Can you work these out from the model? Positions are in its coordinate system, mm. A direction names the side the tool comes from. Coordinates: 2 decimals unless noted, no trailing zeros. Loops run counter-clockwise (first coordinate to the right, second up) from the corner with the lowest first, then second, coordinate; pieces in that order, holes last. Notation, with made-up numbers: (41.5, -32) -> (82.5, -32) arc R10 cw to (82.5, -18) -> close; hole circle Ø5 at (29, -32.75). An arc over 180 degrees is marked (long way). Put each result on its own line as item: value. Start each with the question number.
Item 1: If we section it at A-A on x = 3: Please give me the cut outline in (y, z).
Item 2: If we section it at D-D on y = -0.5: Please give me the cut outline in (x, z), plus the area to 3 significant figures.
Item 3: If we section it at C-C on z = 2.1: Please give me the cut outline in (x, y), plus the area to 3 significant figures.
Item 4: Will these pins go through, and if not, where does the flat tip stop? P1, Ø8, axis at x = 22.45, y = -14.7, coming from the -Z side; P2, Ø6, axis at x = -9, y = -24.5, coming from the -Z side; P3, Ø0.8, axis at y = 21, z = 1.5, coming from the -X side; P4, Ø1, axis at x = -22.5, z = 2, coming from the +Y side.
Item 5: Please list where these lines run through material, in increasing order: L1, parallel to X at y = -2, z = 0.8; L2, parallel to Y at x = -12.5, z = 1.45; L3, parallel to Y at x = -11, z = 1. Write a range as from..to.
Item 6: If we section it at B-B on y = -16: Please give me the cut outline in (x, z), plus the area to 3 significant figures.
Item 7: For faces 1 (the cylindrical face through (-27.35, -3.14, 0.25)), 2 (the flat face through (11.1, 26.1, 1.2)), 3 (the cylindrical face through (2.761, 20.073, 1.232)), 4 (the flat face through (-23, 16.353, 1)), 5 (the cylindrical face through (-5.8, 23.43, 0.49)), which set-ups out of +Z, -Z, +X, -X, +Y, -Y let a thin tool reach every point of the face, with its end or its side?
Item 8: We'd pull the mould along Y, two halves only. Please class faces 6 (the flat face through (22, -28.197, 1)), 7 (the flat face through (4, 28.403, 1)), 8 (the cylindrical face through (20.608, -13.007, 1.486)): pulls with the +Y half, pulls with the -Y half, needs draft (parallel to the pull), parting line crosses it, or undercut.
```python
from build123d import *

# Parameters (mm, degrees)
SKETCH_1_R          = 3
SKETCH_1_R_2        = 2.5
EXTRUDE_1_DEPTH     = 2.5
EXTRUDE_START       = -2
SKETCH_3_R          = 2.5
EXTRUDE_3_DEPTH     = 2
SKETCH_7_R          = 2.65
CUT_EXTRUDE_1_DEPTH = 1
CHAMFER_1_SIZE      = 1
CUT_EXTRUDE_3_REACH = 53.597
SKETCH_10_R         = 2.5
CUT_EXTRUDE_4_REACH = 53.635
CHAMFER_2_SIZE      = 1.5
CUT_EXTRUDE_5_REACH = 53.635
CHAMFER_3_SIZE      = 2
CUT_EXTRUDE_6_REACH = 49.547
SKETCH_15_W         = 9
SKETCH_15_H         = 44.55
SKETCH_15_H_2       = 52
CUT_EXTRUDE_7_REACH = 42.704
SKETCH_16_R         = 2.5
CHAMFER_4_SIZE      = 1.5
SKETCH_17_R         = 2
CUT_EXTRUDE_8_DEPTH = 10


with BuildPart() as part:
    # 스케치1 → 보스-돌출1 (new body)
    with BuildSketch(Plane.XY):
        with BuildLine():
            Line((-27.349187557, -28.196867314), (-7.694270353, -28.196867314))
            Line((-7.694270353, -28.196867314), (-3.192250131, -23.196867314))
            Line((-3.192250131, -23.196867314), (12.267749869, -23.196867314))
            Line((12.267749869, -23.196867314), (17.250812443, -27.683637009))
            Line((17.250812443, -27.683637009), (17.250812443, -14.696867314))
            ThreePointArc((17.250812443, -14.696867314), (22.450812443, -9.496867314), (27.650812443, -14.696867314))
            Line((27.650812443, -14.696867314), (27.650812443, -28.196867314))
            Line((27.650812443, -28.196867314), (40.650812443, -28.196867314))
            Line((40.650812443, -28.196867314), (40.650812443, 12.183132686))
            Line((40.650812443, 12.183132686), (28.992507116, 23.803132686))
            Line((28.992507116, 23.803132686), (13.742507116, 23.803132686))
            Line((13.742507116, 23.803132686), (8.450812443, 28.403132686))
            Line((8.450812443, 28.403132686), (-0.749187557, 28.403132686))
            Line((-0.749187557, 28.403132686), (-5.349187557, 23.803132686))
            Line((-5.349187557, 23.803132686), (-28.149187557, 23.803132686))
            Line((-28.149187557, 23.803132686), (-43.049187557, 8.903132686))
            Line((-43.049187557, 8.903132686), (-43.049187557, -28.196867314))
            Line((-43.049187557, -28.196867314), (-37.749187557, -28.196867314))
            Line((-37.749187557, -28.196867314), (-37.749187557, -3.196867314))
            ThreePointArc((-37.749187557, -3.196867314), (-29.949187557, 1.306464785), (-29.949187557, -7.700199414))
            Line((-29.949187557, -7.700199414), (-29.949187557, -28.196867314))
            Line((-29.949187557, -28.196867314), (-27.349187557, -28.196867314))
        make_face()
        with Locations((8.802507116, -1.986867314)):
            Circle(SKETCH_1_R, mode=Mode.SUBTRACT)
        with Locations((-21.197492884, 7.013132686)):
            Circle(SKETCH_1_R_2, mode=Mode.SUBTRACT)
        with Locations((3.302507116, 22.513132686)):
            Circle(SKETCH_1_R_2, mode=Mode.SUBTRACT)
    extrude(amount=EXTRUDE_1_DEPTH)

    # 스케치3 → 보스-돌출3 (add)
    # profile 1 of 2: a face of its own
    with BuildSketch(Plane.XY.offset(2.5).offset(EXTRUDE_START)):
        with BuildLine():
            Line((27.650812443, -14.696867314), (27.650812443, -28.196867314))
            Line((27.650812443, -28.196867314), (17.764042748, -28.196867314))
            Line((17.764042748, -28.196867314), (17.250812443, -27.683637009))
            Line((17.250812443, -27.683637009), (17.250812443, -14.696867314))
            ThreePointArc((17.250812443, -14.696867314), (22.450812443, -9.496867314), (27.650812443, -14.696867314))
        make_face()
        with Locations((22.450812443, -14.696867314)):
            Circle(SKETCH_3_R, mode=Mode.SUBTRACT)
    # profile 2 of 2: a face of its own
    with BuildSketch(Plane.XY.offset(2.5).offset(EXTRUDE_START)):
        with BuildLine():
            Line((-29.949187557, -7.700199414), (-29.949187557, -28.196867314))
            Line((-29.949187557, -28.196867314), (-30.049187557, -28.196867314))
            Line((-30.049187557, -28.196867314), (-37.749187557, -28.196867314))
            Line((-37.749187557, -28.196867314), (-37.749187557, -3.196867314))
            ThreePointArc((-37.749187557, -3.196867314), (-29.949187557, 1.306464785), (-29.949187557, -7.700199414))
        make_face()
        with Locations((-32.549187557, -3.196867314)):
            Circle(SKETCH_3_R, mode=Mode.SUBTRACT)
    extrude(amount=EXTRUDE_3_DEPTH)

    # 스케치7 → 컷-돌출1 (cut)
    with BuildSketch(Plane(origin=(0, 0, 0), x_dir=(-1, 0, 0), z_dir=(0, 0, -1))):
        with Locations((6.149187557, 20.803132686)):
            Circle(SKETCH_7_R)
        with Locations((8.049187557, -24.196867314)):
            Circle(SKETCH_7_R)
        with BuildLine():
            Line((-26.406412787, 7.908733029), (-32.895212099, 7.908733029))
            ThreePointArc((-32.895212099, 7.908733029), (-33.708384897, 8.245560231), (-34.045212099, 9.058733029))
            Line((-34.045212099, 9.058733029), (-34.045212099, 15.547532342))
            ThreePointArc((-34.045212099, 15.547532342), (-33.708384897, 16.36070514), (-32.895212099, 16.697532342))
            Line((-32.895212099, 16.697532342), (-29.650812443, 16.697532342))
            ThreePointArc((-29.650812443, 16.697532342), (-26.543502647, 15.410442482), (-25.256412787, 12.303132686))
            Line((-25.256412787, 12.303132686), (-25.256412787, 9.058733029))
            ThreePointArc((-25.256412787, 9.058733029), (-25.593239988, 8.245560231), (-26.406412787, 7.908733029))
        make_face()
    extrude(amount=-CUT_EXTRUDE_1_DEPTH, mode=Mode.SUBTRACT)

    # 모따기1
    chamfer_1_edges = [part.edges().sort_by_distance(p)[0] for p in [
        (-43.049187557, -28.196867314, 1.25),
        (40.650812443, -28.196867314, 1.25),
    ]]
    chamfer(chamfer_1_edges, length=CHAMFER_1_SIZE)

    # 스케치10 → 컷-돌출3 (cut, up to next)
    with BuildSketch(Plane(origin=(0, 0, 1), x_dir=(-1, 0, 0), z_dir=(0, 0, -1)), mode=Mode.PRIVATE) as cut_extrude_3_sk1:
        with Locations((-29.650812443, 12.303132686)):
            Circle(SKETCH_10_R)
    cut_extrude_3_tool1 = extrude(cut_extrude_3_sk1.sketch, amount=-CUT_EXTRUDE_3_REACH, mode=Mode.PRIVATE) & part.part
    add(cut_extrude_3_tool1.solids().sort_by_distance((29.650812, 12.303133, 1))[0], mode=Mode.SUBTRACT)

    # 스케치12 → 컷-돌출4 (cut, up to next)
    with BuildSketch(Plane(origin=(0, 0, 0), x_dir=(-1, 0, 0), z_dir=(0, 0, -1)), mode=Mode.PRIVATE) as cut_extrude_4_sk1:
        Polygon((16.749187557, 23.803132686), (16.749187557, 16.353132686), (35.599187557, 16.353132686), (28.149187557, 23.803132686), align=None)
    cut_extrude_4_tool1 = extrude(cut_extrude_4_sk1.sketch, amount=-CUT_EXTRUDE_4_REACH, mode=Mode.PRIVATE) & part.part
    add(cut_extrude_4_tool1.solids().sort_by_distance((-24.464587, 19.772334, 0))[0], mode=Mode.SUBTRACT)

    # 모따기2
    chamfer_2_edges = [part.edges().sort_by_distance(p)[0] for p in [
        (-16.749187557, 23.803132686, 1.25),
        (-16.749187557, 16.353132686, 1.25),
    ]]
    chamfer(chamfer_2_edges, length=CHAMFER_2_SIZE)

    # 스케치13 → 컷-돌출5 (cut, up to next)
    with BuildSketch(Plane(origin=(0, 0, 0), x_dir=(-1, 0, 0), z_dir=(0, 0, -1)), mode=Mode.PRIVATE) as cut_extrude_5_sk1:
        Polygon((-34.689283113, 18.125074406), (-34.689283113, -28.196867314), (-39.650812443, -28.196867314), (-40.650812443, -27.196867314), (-40.650812443, 12.183132686), align=None)
    cut_extrude_5_tool1 = extrude(cut_extrude_5_sk1.sketch, amount=-CUT_EXTRUDE_5_REACH, mode=Mode.PRIVATE) & part.part
    # 스케치13 → 컷-돌출5 (cut, up to next)
    with BuildSketch(Plane(origin=(0, 0, 0), x_dir=(-1, 0, 0), z_dir=(0, 0, -1)), mode=Mode.PRIVATE) as cut_extrude_5_sk2:
        Polygon((38.049187557, 13.903132686), (43.049187557, 8.903132686), (43.049187557, -27.196867314), (42.049187557, -28.196867314), (38.049187557, -28.196867314), align=None)
    cut_extrude_5_tool2 = extrude(cut_extrude_5_sk2.sketch, amount=-CUT_EXTRUDE_5_REACH, mode=Mode.PRIVATE) & part.part
    add(cut_extrude_5_tool1.solids().sort_by_distance((37.59669, -6.446011, 0))[0], mode=Mode.SUBTRACT)
    add(cut_extrude_5_tool2.solids().sort_by_distance((-40.49096, -8.321213, 0))[0], mode=Mode.SUBTRACT)

    # 모따기3
    chamfer_3_edges = [part.edges().sort_by_distance(p)[0] for p in [
        (-38.049187557, -28.196867314, 1.25),
        (34.689283113, -28.196867314, 1.25),
    ]]
    chamfer(chamfer_3_edges, length=CHAMFER_3_SIZE)

    # 스케치15 → 컷-돌출6 (cut, up to next)
    with BuildSketch(Plane.XY.offset(2.5), mode=Mode.PRIVATE) as cut_extrude_6_sk1:
        with Locations((-33.549187557, -5.921867314)):
            Rectangle(SKETCH_15_W, SKETCH_15_H)
    cut_extrude_6_tool1 = extrude(cut_extrude_6_sk1.sketch, amount=-CUT_EXTRUDE_6_REACH, mode=Mode.PRIVATE) & part.part
    # 스케치15 → 컷-돌출6 (cut, up to next)
    with BuildSketch(Plane.XY.offset(2.5), mode=Mode.PRIVATE) as cut_extrude_6_sk2:
        with Locations((30.189283113, -2.196867314)):
            Rectangle(SKETCH_15_W, SKETCH_15_H_2)
    cut_extrude_6_tool2 = extrude(cut_extrude_6_sk2.sketch, amount=-CUT_EXTRUDE_6_REACH, mode=Mode.PRIVATE) & part.part
    add(cut_extrude_6_tool1.solids().sort_by_distance((-33.549188, -5.921867, 2.5))[0], mode=Mode.SUBTRACT)
    add(cut_extrude_6_tool2.solids().sort_by_distance((30.189283, -2.196867, 2.5))[0], mode=Mode.SUBTRACT)

    # 스케치16 → 컷-돌출7 (cut, up to next)
    with BuildSketch(Plane(origin=(0, 0, 0), x_dir=(-1, 0, 0), z_dir=(0, 0, -1)), mode=Mode.PRIVATE) as cut_extrude_7_sk1:
        with Locations((11.549187557, -2.196867314)):
            Circle(SKETCH_16_R)
    cut_extrude_7_tool1 = extrude(cut_extrude_7_sk1.sketch, amount=-CUT_EXTRUDE_7_REACH, mode=Mode.PRIVATE) & part.part
    add(cut_extrude_7_tool1.solids().sort_by_distance((-11.549188, -2.196867, 0))[0], mode=Mode.SUBTRACT)

    # 모따기4
    chamfer_4_edges = [part.edges().sort_by_distance(p)[0] for p in [
        (-29.049187557, 16.353132686, 1.25),
        (-29.049187557, -28.196867314, 1.25),
    ]]
    chamfer(chamfer_4_edges, length=CHAMFER_4_SIZE)

    # 스케치17 → 컷-돌출8 (cut)
    with BuildSketch(Plane(origin=(0, 0, 0), x_dir=(-1, 0, 0), z_dir=(0, 0, -1))):
        with Locations((11.219187557, 20.503132686)):
            Circle(SKETCH_17_R)
    extrude(amount=-CUT_EXTRUDE_8_DEPTH, mode=Mode.SUBTRACT)


solid = part.part
```
Solutions:
1. outline: (-23.2, 0) -> (20.03, 0) -> (20.03, 2.5) -> (-23.2, 2.5) -> close; (24.99, 0) -> (28.4, 0) -> (28.4, 2.5) -> (24.99, 2.5) -> close
2. outline: (-29.05, 0.5) -> (-28.1, 0.5) -> (-28.1, 0) -> (-13.39, 0) -> (-13.39, 2.5) -> (-29.05, 2.5) -> close; (-9.71, 0) -> (6.2, 0) -> (6.2, 2.5) -> (-9.71, 2.5) -> close; (11.41, 0) -> (25.69, 0) -> (25.69, 2.5) -> (11.41, 2.5) -> close
2. area: 114 mm^2
3. outline: (-29.05, -26.7) -> (-27.55, -28.2) -> (-7.69, -28.2) -> (-3.19, -23.2) -> (12.27, -23.2) -> (17.25, -27.68) -> (17.76, -28.2) -> (25.69, -28.2) -> (25.69, 23.8) -> (13.74, 23.8) -> (8.45, 28.4) -> (-0.75, 28.4) -> (-5.35, 23.8) -> (-15.25, 23.8) -> (-16.75, 22.3) -> (-16.75, 17.85) -> (-18.25, 16.35) -> (-27.55, 16.35) -> (-29.05, 14.85) -> close; hole circle Ø5 at (-21.2, 7.01); hole circle Ø5 at (-11.55, -2.2); hole circle Ø4 at (-11.22, 20.5); hole circle Ø5 at (3.3, 22.51); hole circle Ø6 at (8.8, -1.99); hole circle Ø5 at (22.45, -14.7)
3. area: 2,600 mm^2
4. P1: z = 0.5
4. P2: z = 0
4. P3: x = -16.75
4. P4: y = 16.35
5. L1: -29.05..-14.04, -9.06..5.8, 11.8..25.69
5. L2: -28.2..-4.51, 0.12..18.97, 22.04..23.8
5. L3: -28.2..-4.64, 0.24..18.52, 22.49..23.8
6. outline: (-29.05, 0) -> (17.25, 0) -> (17.25, 0.5) -> (20.32, 0.5) -> (20.32, 2.5) -> (-29.05, 2.5) -> close; (24.58, 0.5) -> (25.69, 0.5) -> (25.69, 2.5) -> (24.58, 2.5) -> close
6. area: 124 mm^2
7. face 1: -Z, -X
7. face 2: +Z, -Z, +X, +Y
7. face 3: +Z, -Z
7. face 4: +Z, -Z, -X, +Y
7. face 5: -Z
8. face 6: pulls with the -Y half
8. face 7: pulls with the +Y half
8. face 8: undercut
